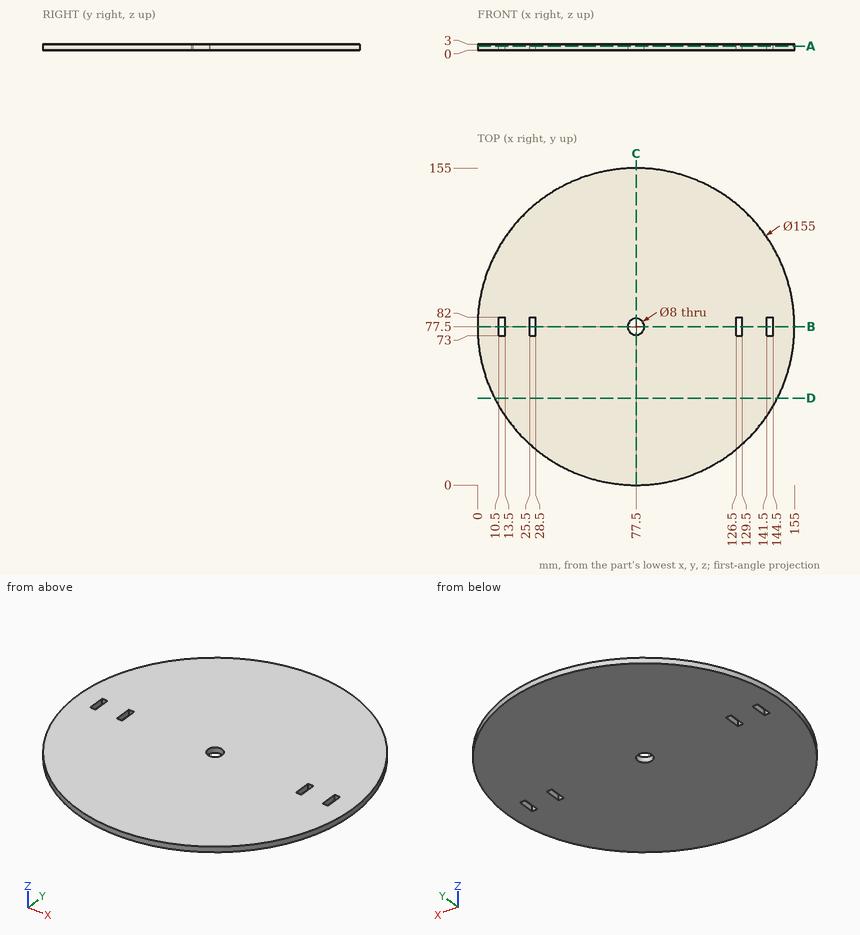
Input: dimensioned drawing with shaded views. Units: mm. Origin: part minimum x, y, z. Round coordinates to 2 decimals unless told otherwise and drop trailing zeros. Order: outer loops, then holes, each group sorted by start corner. A loop starts at its lowest first (then second) coordinate and runs counter-clockwise, first axis right, second up. Notation, with made-up numbers: (82.25, 31) -> (133.25, 31) arc R23 cw to (133.25, 40) -> close; hole circle Ø8 at (89, 87.25). An arc over 180 degrees is marked (long way). One line per item, written item: value. Start each with the question number.
Q1. Section query A-A (z = 2). Return the cut outline in (x, y).
Q2. Section query C-C (x = 77.5). Return the cut outline in (y, z), plus the area to 3 significant figures.
Q3. Material intervals for probe 1 along X at (y, z) = (80, 0.95); probe 2 along Y at (x, z) = (77.5, 1.7); probe 3 along Y at (x, z) = (75, 1.25), sorted ascending.
Q4. Section query B-B (y = 77.5). Return the cut outline in (x, z).
Q5. Section query D-D (y = 42.5). Return the cut outline in (x, z).
Q6. Pin query (flat end, axial travel): pin 1 (0.9 mm diameter, centred on y = 78, z = 1.5, fed in from -X); pin 2 (1.5 mm diameter, centred on x = 12.5, z = 2, fed in from +Y); pin 3 (1.5 mm diameter, centred on x = 11.5, z = 1.5, fed in from -Y); pin 4 (0.9 mm diameter, centred on x = 27, z = 2, fed in from -Y). Return the tip coordinate at first contact, or that it passes through.
Findings below:
1. outline: circle Ø155 at (77.5, 77.5); hole (10.5, 73) -> (13.5, 73) -> (13.5, 82) -> (10.5, 82) -> close; hole (25.5, 73) -> (28.5, 73) -> (28.5, 82) -> (25.5, 82) -> close; hole circle Ø8 at (77.5, 77.5); hole (126.5, 73) -> (129.5, 73) -> (129.5, 82) -> (126.5, 82) -> close; hole (141.5, 73) -> (144.5, 73) -> (144.5, 82) -> (141.5, 82) -> close
2. outline: (0, 0) -> (73.5, 0) -> (73.5, 3) -> (0, 3) -> close; (81.5, 0) -> (155, 0) -> (155, 3) -> (81.5, 3) -> close
2. area: 441 mm²
3. probe 1: 0.04 to 10.5, 13.5 to 25.5, 28.5 to 74.38, 80.62 to 126.5, 129.5 to 141.5, 144.5 to 154.96
3. probe 2: 0 to 73.5, 81.5 to 155
3. probe 3: 0.04 to 74.38, 80.62 to 154.96
4. outline: (0, 0) -> (10.5, 0) -> (10.5, 3) -> (0, 3) -> close; (13.5, 0) -> (25.5, 0) -> (25.5, 3) -> (13.5, 3) -> close; (28.5, 0) -> (73.5, 0) -> (73.5, 3) -> (28.5, 3) -> close; (81.5, 0) -> (126.5, 0) -> (126.5, 3) -> (81.5, 3) -> close; (129.5, 0) -> (141.5, 0) -> (141.5, 3) -> (129.5, 3) -> close; (144.5, 0) -> (155, 0) -> (155, 3) -> (144.5, 3) -> close
5. outline: (8.35, 0) -> (146.65, 0) -> (146.65, 3) -> (8.35, 3) -> close
6. pin 1: x = 0
6. pin 2: y = 120.84
6. pin 3: y = 35.68
6. pin 4: y = 18.33
